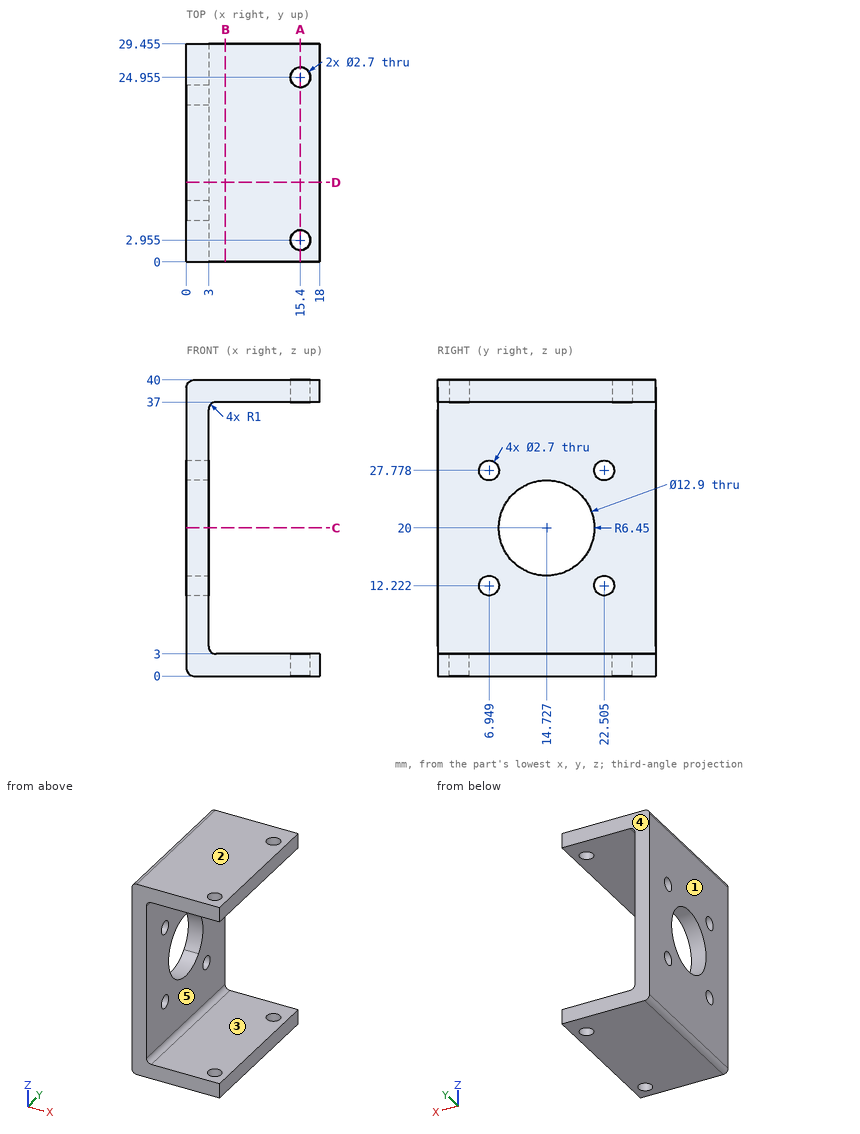
Drawing for the job (mm, zero at the part's lowest x, y, z). A direction names the side the tool comes from. Round coordinates to 2 decimals unless told otherwise and drop trailing zeros. Write each loop counter-clockwise with the first axis right and the second up, starting at its lowest first coordinate (ties: lowest second). Pieces come first, ordered by that corner, then holes.
Item 1: Band-saw the part on A-A on x = 15.4. Write the cut outline in (y, z) (1 decimal), then the cut area to 3 significant figures.
Filled in:
outline: (0, 0) - (1.6, 0) - (1.6, 3) - (0, 3) - close; (0, 37) - (1.6, 37) - (1.6, 40) - (0, 40) - close; (4.3, 0) - (23.6, 0) - (23.6, 3) - (4.3, 3) - close; (4.3, 37) - (23.6, 37) - (23.6, 40) - (4.3, 40) - close; (26.3, 0) - (29.5, 0) - (29.5, 3) - (26.3, 3) - close; (26.3, 37) - (29.5, 37) - (29.5, 40) - (26.3, 40) - close
area: 144 mm2
Item 2: Drop a flat-ended pin along its axis: pin 1 Ø14.5 at (y, z) = (14, 22.5) entering from +X. Give the stop position or say it passes through.
Filled in:
pin 1: stops at x = 3
Item 3: Band-saw the part on C-C on z = 20. Write the cut outline in (x, y) (1 decimal).
Filled in:
outline: (0, 0) - (3, 0) - (3, 8.3) - (0, 8.3) - close; (0, 21.2) - (3, 21.2) - (3, 29.5) - (0, 29.5) - close
Item 4: Band-saw the part on D-D on y = 10.75. Write the cut outline in (x, z).
Filled in:
outline: (0, 1) arc R1 ccw to (1, 0) - (18, 0) - (18, 3) - (4, 3) arc R1 cw to (3, 4) - (3, 14.92) - (0, 14.92) - close; (0, 25.08) - (3, 25.08) - (3, 36) arc R1 cw to (4, 37) - (18, 37) - (18, 40) - (1, 40) arc R1 ccw to (0, 39) - close
Item 5: Mould opens along Z. For the marked faces 1, 2 and 3 say: released by +Z, released by -Z, zero draft, split by the parting line, or undercut.
Filled in:
face 1: zero draft
face 2: released by +Z
face 3: undercut
Item 6: Tool access for the marked faces 4 and 5: list every direction of +Z, -Z, +X, -X, +Y, -Y with a clear straight run to the whole face (end or side of a thin tool).
Filled in:
face 4: +Z, -Z, +X, -X, +Y
face 5: +X, +Y, -Y
Item 7: Drill centre lines: L1, parallel to Y at x = 15.4, z = 38.95 (1 decimal); L2, parallel to Z at x = 13, y = 18.75; L3, parallel to Y at x = 1.35, z = 20 (1 decimal). Where is each one in solid material? Low to high.
Filled in:
L1: y = 0 to 1.6, 4.3 to 23.6, 26.3 to 29.5
L2: z = 0 to 3, 37 to 40
L3: y = 0 to 8.3, 21.2 to 29.5
Item 8: Band-saw the part on B-B on x = 5.25. Write the cut outline in (y, z) (1 decimal), then the cut area to 3 significant figures.
Filled in:
outline: (0, 0) - (29.5, 0) - (29.5, 3) - (0, 3) - close; (0, 37) - (29.5, 37) - (29.5, 40) - (0, 40) - close
area: 177 mm2
